Input: dimensioned drawing with shaded views. Units: mm. Origin: part minimum x, y, z. Round coordinates to 2 decimals unless told otherwise and drop trailing zeros. Order: outer loops, then holes, each group sorted by start corner. A loop starts at its lowest first (then second) coordinate and runs counter-clockwise, first axis right, second up.
Item 1: First-contact query: pin 1 (1.5 mm diameter, centred on x = 71, y = 0.5, fed in from +Z) (1 decimal); pin 2 (0.9 mm diameter, centred on x = 40.5, y = 2, fed in from -Z). Flat tips, straight axial feed; report the tip coordinate or a pass-through.
Item 2: Cut plane A-A on x = 91. Output: boundary loops of the cut face in (y, z) (1 decimal), then the cut area to 3 significant figures.
Item 3: Cut plane B-B on z = 16.5. Output: boundary loops of the cut face in (x, y) (1 decimal).
Item 4: Cut plane D-D on y = 0.6. Output: boundary loops of the cut face in (x, z) (1 decimal).
Item 5: Cut plane C-C on z = 3. Output: boundary loops of the cut face in (x, y) (1 decimal).
Item 6: Line query: L1, parallel to X at y = 2.3, z = 3 (1 decimal); L2, parallel to Z at x = 44, y = 0.15 (1 decimal); L3, parallel to X at y = 0.1, z = 49 (1 decimal). Output: solid intervals per line, ascending.
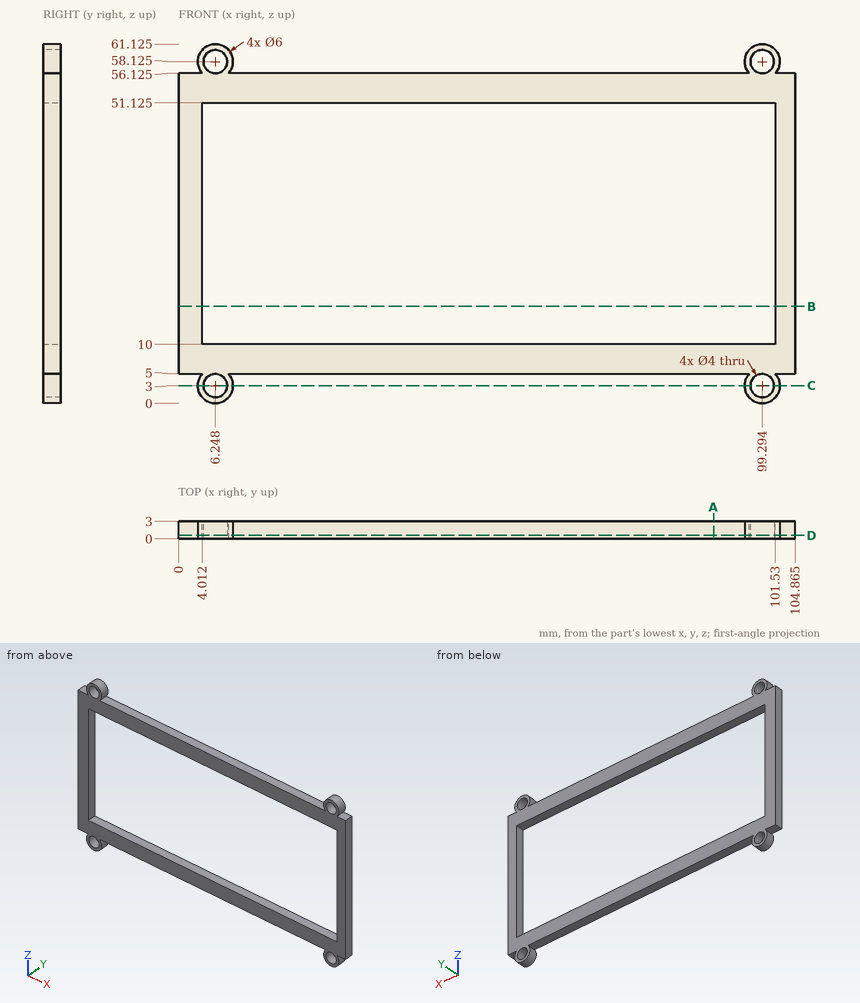
From the geometry:
1. pin 1: stops at z = 56.1
1. pin 2: stops at z = 5
2. outline: (0, 5) - (3, 5) - (3, 10) - (0, 10) - close; (0, 51.1) - (3, 51.1) - (3, 56.1) - (0, 56.1) - close
2. area: 30.0 mm2
3. outline: (0, 0) - (4, 0) - (4, 3) - (0, 3) - close; (101.5, 0) - (104.9, 0) - (104.9, 3) - (101.5, 3) - close
4. outline: (0, 5) - (4, 5) arc R3 ccw (long way) to (8.5, 5) - (97.1, 5) arc R3 ccw (long way) to (101.5, 5) - (104.9, 5) - (104.9, 56.1) - (101.5, 56.1) arc R3 ccw (long way) to (97.1, 56.1) - (8.5, 56.1) arc R3 ccw (long way) to (4, 56.1) - (0, 56.1) - close; hole (4, 10) - (101.5, 10) - (101.5, 51.1) - (4, 51.1) - close; hole circle Ø4 at (6.2, 3); hole circle Ø4 at (6.2, 58.1); hole circle Ø4 at (99.3, 3); hole circle Ø4 at (99.3, 58.1)
5. outline: (3.2, 0) - (4.2, 0) - (4.2, 3) - (3.2, 3) - close; (8.2, 0) - (9.2, 0) - (9.2, 3) - (8.2, 3) - close; (96.3, 0) - (97.3, 0) - (97.3, 3) - (96.3, 3) - close; (101.3, 0) - (102.3, 0) - (102.3, 3) - (101.3, 3) - close
6. L1: x = 3.2 to 4.2, 8.2 to 9.2, 96.3 to 97.3, 101.3 to 102.3
6. L2: z = 5 to 10, 51.1 to 56.1
6. L3: x = 0 to 4, 101.5 to 104.9
